Could you check a few things on this drawing? It's one solid part, dimensions in mm from its lowest x, y, z. Coordinates: 2 decimals unless noted, no trailing zeros. Write each loop counter-clockwise with the first axis right and the second up, starting at its lowest first coordinate (ties: lowest second). Pieces come first, ordered by that corner, then holes. Notation, with made-up numbers: M -16.75,3 L 25.25,3 A20 ccw 25.25,30 Z; hole C 3.5,-29.5 d2. An arc over 180 degrees is marked long. Use a Markdown table: item, result.
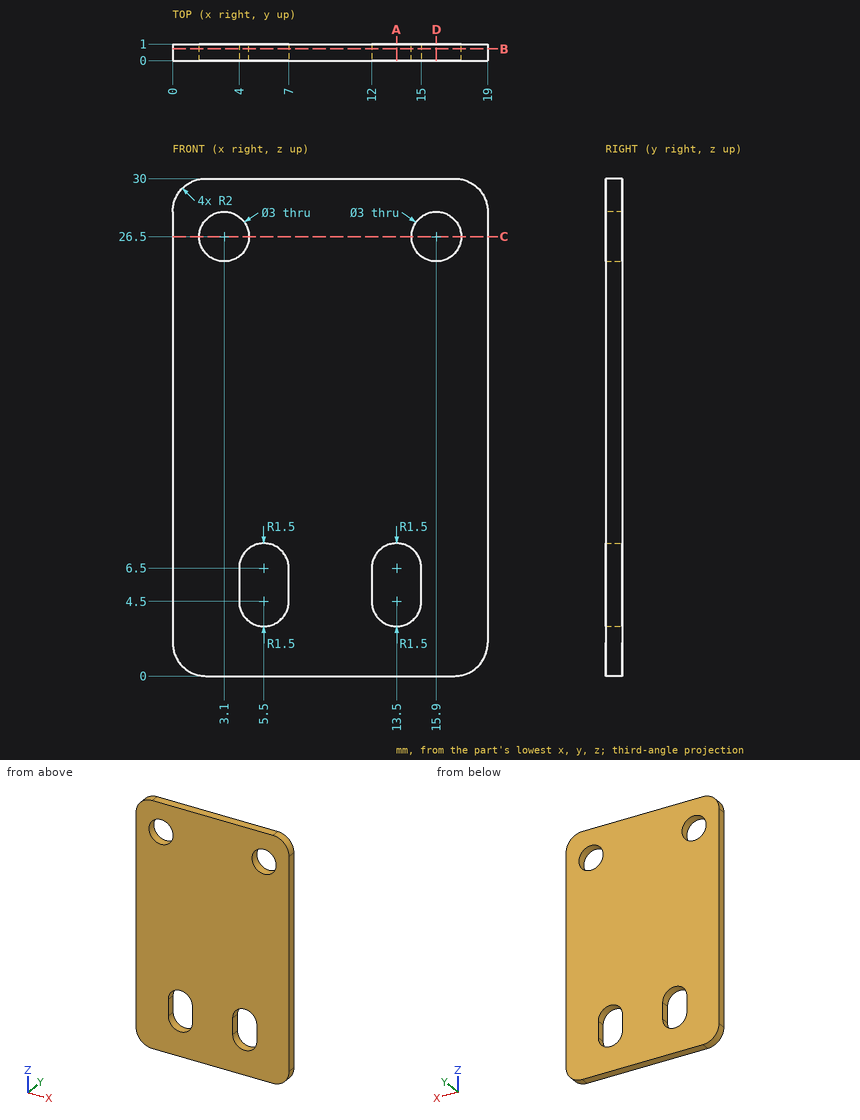
1. I need wall thicknesses on probe 1 along X at (y, z) = (0.5, 26.5); probe 2 along Z at (x, y) = (3, 0.55); probe 3 along Z at (x, y) = (6.75, 0.3). Which ranges of each line are inside material? Lowest first, please.
Answers follow:
| item | result |
|---|---|
| probe 1 | x = 0 to 1.6, 4.6 to 14.4, 17.4 to 19 |
| probe 2 | z = 0 to 25, 28 to 30 |
| probe 3 | z = 0 to 3.67, 7.33 to 30 |
2. Suppose I cut it at D-D on x = 15.9. Write out the boundary of the cut face in (y, z), and give its area (3 significant figures).
Answers follow:
| item | result |
|---|---|
| outline | M 0,0 L 1,0 L 1,25 L 0,25 Z; M 0,28 L 1,28 L 1,30 L 0,30 Z |
| area | 27.0 mm2 |
3. Suppose I cut it at A-A on x = 13.5. Write out the boundary of the cut face in (y, z).
Answers follow:
| item | result |
|---|---|
| outline | M 0,0 L 1,0 L 1,3 L 0,3 Z; M 0,8 L 1,8 L 1,30 L 0,30 Z |
4. Suppose I cut it at B-B on y = 0.7. Write out the boundary of the cut face in (x, z).
Answers follow:
| item | result |
|---|---|
| outline | M 0,2 A2 ccw 2,0 L 17,0 A2 ccw 19,2 L 19,28 A2 ccw 17,30 L 2,30 A2 ccw 0,28 Z; hole C 3.1,26.5 d3; hole M 4,4.5 A1.5 ccw 7,4.5 L 7,6.5 A1.5 ccw 4,6.5 Z; hole M 12,4.5 A1.5 ccw 15,4.5 L 15,6.5 A1.5 ccw 12,6.5 Z; hole C 15.9,26.5 d3 |
5. Suppose I cut it at C-C on z = 26.5. Write out the boundary of the cut face in (x, y).
Answers follow:
| item | result |
|---|---|
| outline | M 0,0 L 1.6,0 L 1.6,1 L 0,1 Z; M 4.6,0 L 14.4,0 L 14.4,1 L 4.6,1 Z; M 17.4,0 L 19,0 L 19,1 L 17.4,1 Z |
